from build123d import *

# Parameters (mm, degrees)
F1_DEPTH = 50.8
F2_R     = 1.5875
F3_DEPTH = 5.715
F4_SIZE  = 5.08
F6_DEPTH = 50.8


with BuildPart() as f1:
    # F0 (on Front) → F1 (new body)
    with BuildSketch(Plane.XZ):
        Polygon((25.4, 57.785), (25.4, 63.5), (0, 63.5), (0, 0), (50.8, 0), (101.6, 0), (101.6, 63.5), (76.2, 63.5), (76.2, 57.785), (88.9, 57.785), (88.9, 53.975), (76.2, 53.975), (76.2, 48.26), (88.9, 48.26), (88.9, 10.16), (50.8, 10.16), (12.7, 10.16), (12.7, 48.26), (25.4, 48.26), (25.4, 53.975), (12.7, 53.975), (12.7, 57.785), align=None)
    extrude(amount=F1_DEPTH)

    # F2 (on face) → F3 (cut, through all)
    with BuildSketch(Plane.XY.offset(63.5)):
        with Locations((19.05, -25.4)):
            Circle(F2_R)
        with Locations((82.55, -25.4)):
            Circle(F2_R)
    extrude(amount=-F3_DEPTH, mode=Mode.SUBTRACT)

    # F4
    f4_edges = [f1.edges().sort_by_distance(p)[0] for p in [
        (12.7, -25.4, 10.16),
        (88.9, -25.4, 10.16),
        (12.7, -25.4, 48.26),
        (88.9, -25.4, 48.26),
    ]]
    chamfer(f4_edges, length=F4_SIZE)

    # F5 (on face) → F6 (join)
    with BuildSketch(Plane.XZ.offset(50.8)):
        Polygon((0, 47.963981), (0, 63.5), (-4.432204, 63.5), align=None)
        Polygon((101.6, 63.5), (101.6, 47.963981), (106.032204, 63.5), align=None)
    extrude(amount=-F6_DEPTH)


solid = f1.part
Design review of the part built by this model. Coordinates are the model's own, in mm. A direction names the side the tool comes from. Coordinates: 2 decimals unless noted, no trailing zeros. Loops run counter-clockwise (first coordinate to the right, second up) from the corner with the lowest first, then second, coordinate; pieces in that order, holes last. Notation, with made-up numbers: M 81.25,48.5 L 113.25,48.5 A29 cw 113.25,79.5 Z; hole C -20.75,76.25 d9. An arc over 180 degrees is marked long. Answer as CSV lines item,"result".
Item 1: Machinability: for faces 4 (the face through (12.7, -25, 56)), 5 (the face through (50, -50.8, 4)), 6 (the face through (76.2, -25, 61)), 7 (the face through (91, -25, 63.5)), 8 (the face through (83.4, -24.06, 60.68)), which of the approach directions +Z, -Z, +X, -X, +Y, -Y give a long, thin tool a straight path to every point of the face, cutting with its end or side? Answer none if there is none.
Answer list:
face 4,"+Y, -Y"
face 5,"+Z, -Z, +X, -X, -Y"
face 6,"+Z, +Y, -Y"
face 7,"+Z, +X, -X, +Y, -Y"
face 8,"+Z"
Item 2: Add section C-C on x = 87.5. State the section outline as (y, z) points (3 decimals), plus the area to 3 significant figures.
Answer list:
outline,"M -50.8,0 L 0,0 L 0,13.84 L -50.8,13.84 Z; M -50.8,44.58 L 0,44.58 L 0,53.975 L -50.8,53.975 Z; M -50.8,57.785 L 0,57.785 L 0,63.5 L -50.8,63.5 Z"
area,"1,470 mm²"
Item 3: Add section D-D on x = 19.05. State the section outline as (y, z) points (1 decimal), plus the area to 3 significant figures.
Answer list:
outline,"M -50.8,0 L 0,0 L 0,10.2 L -50.8,10.2 Z; M -50.8,48.3 L 0,48.3 L 0,54 L -50.8,54 Z; M -50.8,57.8 L -27,57.8 L -27,63.5 L -50.8,63.5 Z; M -23.8,57.8 L 0,57.8 L 0,63.5 L -23.8,63.5 Z"
area,"1,080 mm²"
Item 4: For P1, Ø4.5, axis at y = -23, z = 50.5, coming from the +X side; P2, Ø4.5, axis at y = -20, z = 51.5, coming from the -X side; P3, Ø3, axis at y = -19, z = 10, coming from the -X side, all flat-tipped, find the tip position at first contact; note any pin that passes through.
Answer list:
P1,"x = 102.97"
P2,"x = -1.65"
P3,"x = 0"
Item 5: The part is to be moulded in two halves that separate along Y. For faces 1 (the face through (85, -25, 57.785)), 2 (the face through (50, 0, 4)), 3 (the face through (18.843, -23.826, 60.683)), say which applies: pulls with the +Y half, pulls with the -Y half, needs draft (parallel to the pull), parting line crosses it, or undercut.
Answer list:
face 1,"needs draft"
face 2,"pulls with the +Y half"
face 3,"undercut"
Item 6: Add section A-A on y = -25.4. Count the separate pieces of the cut face and the enclosed holes in it, plus the area to 3 significant figures.
Answer list:
separate pieces,"3"
enclosed holes,"0"
area,"2,760 mm²"
Item 7: Add section B-B on z = 27. State the section outline as (x, y) points, plus the area to 3 significant figures.
Answer list:
outline,"M 0,-50.8 L 12.7,-50.8 L 12.7,0 L 0,0 Z; M 88.9,-50.8 L 101.6,-50.8 L 101.6,0 L 88.9,0 Z"
area,"1,290 mm²"
Item 8: For probe 1 along Z at (x, y) = (78.5, -33) (3 decimals); probe 2 along X at (y, z) = (-15, 19); probe 3 along X at (y, z) = (-25, 61), list the stretches that pass through material, from the lowest coordinate up.
Answer list:
probe 1,"0 to 10.16, 48.26 to 53.975, 57.785 to 63.5"
probe 2,"0 to 12.7, 88.9 to 101.6"
probe 3,"-3.72 to 17.51, 20.59 to 25.4, 76.2 to 81.01, 84.09 to 105.32"
